from build123d import *

# Parameters (mm, degrees)
SKETCH1_W           = 260
SKETCH1_H           = 150
BOSS_EXTRUDE1_DEPTH = 15
SKETCH3_R           = 5
CUT_EXTRUDE1_DEPTH  = 16
SKETCH4_R           = 5
CUT_EXTRUDE2_DEPTH  = 16


with BuildPart() as part:
    # Sketch1 → Boss-Extrude1 (new body)
    with BuildSketch(Plane(origin=(0, 0, 0), x_dir=(0, 0, -1), z_dir=(1, 0, 0))):
        Rectangle(SKETCH1_W, SKETCH1_H)
    extrude(amount=BOSS_EXTRUDE1_DEPTH)

    # Sketch3 → Cut-Extrude1 (cut, through all)
    with BuildSketch(Plane.ZY):
        with Locations((0, 55)):
            Circle(SKETCH3_R)
    extrude(amount=-CUT_EXTRUDE1_DEPTH, mode=Mode.SUBTRACT)

    # Sketch4 → Cut-Extrude2 (cut, through all)
    with BuildSketch(Plane.ZY):
        with Locations((-120, 55)):
            Circle(SKETCH4_R)
        with Locations((-117.956771962, 32.950057862)):
            Circle(SKETCH4_R)
        with Locations((-111.896667529, 11.651000058)):
            Circle(SKETCH4_R)
        with Locations((-102.026056288, -8.171859545)):
            Circle(SKETCH4_R)
        with Locations((-88.681070066, -25.843477238)):
            Circle(SKETCH4_R)
        with Locations((-72.316156366, -40.762067274)):
            Circle(SKETCH4_R)
        with Locations((-53.488602693, -52.419594963)):
            Circle(SKETCH4_R)
        with Locations((-32.839558809, -60.419077181)):
            Circle(SKETCH4_R)
        with Locations((-11.072203136, -64.488101155)):
            Circle(SKETCH4_R)
        with Locations((11.072203136, -64.488101155)):
            Circle(SKETCH4_R)
        with Locations((32.839558809, -60.419077181)):
            Circle(SKETCH4_R)
        with Locations((53.488602693, -52.419594963)):
            Circle(SKETCH4_R)
        with Locations((72.316156366, -40.762067274)):
            Circle(SKETCH4_R)
        with Locations((88.681070066, -25.843477238)):
            Circle(SKETCH4_R)
        with Locations((102.026056288, -8.171859545)):
            Circle(SKETCH4_R)
        with Locations((111.896667529, 11.651000058)):
            Circle(SKETCH4_R)
        with Locations((117.956771962, 32.950057862)):
            Circle(SKETCH4_R)
        with Locations((120, 55)):
            Circle(SKETCH4_R)
    extrude(amount=-CUT_EXTRUDE2_DEPTH, mode=Mode.SUBTRACT)


solid = part.part
Geometry check sheet. Reference: the model listing, model coordinates, mm. Round coordinates to 2 decimals unless told otherwise and drop trailing zeros. Loops run counter-clockwise (first coordinate to the right, second up) from the corner with the lowest first, then second, coordinate; pieces in that order, holes last.
Item 1: Cross-section at D-D on x = 2.5. Count the separate pieces of the cut face and the enclosed holes in it, then the cut area to 3 significant figures.
Item 2: Cross-section at C-C on z = 0. Record the boundary of the cut face in (x, y), then the cut area to 3 significant figures.
Item 3: Gauge pin test, flat end, axial feed: pin 1 (11.5 mm diameter, centred on y = -40.76, z = -72.32, fed in from -X). Record the tip position at first contact, or that the pin passes through.
Item 4: Cross-section at B-B on z = -120. Record the boundary of the cut face in (x, y), then the cut area to 3 significant figures.
Item 5: Thickness scan on line 1 (Z direction, x = 4.5, y = 12); line 2 (Z direction, x = 6.5, y = -41); line 3 (Y direction, x = 1.5, z = 116.5). Record the ranges inside material, lowest first.
Item 6: Mould release check, pull along Z, two halves, no side actions. Record for faces 1 (the cylindrical face through (7.4, -69.37, 9.99)), 2 (the flat face through (7, -1, -130)), 3 (the flat face through (7, 75, 2)), 4 (the cylindrical face through (7.395, 59.957, -0.651)): pulls with the +Z half, pulls with the -Z half, needs draft (parallel to the pull), parting line crosses it, or undercut.
Item 7: Cross-section at A-A on y = 55. Record the boundary of the cut face in (x, z), then the cut area to 3 significant figures.
Answer sheet:
1. separate pieces: 1
1. enclosed holes: 19
1. area: 37,500 mm2
2. outline: (0, -75) - (15, -75) - (15, 50) - (0, 50) - close; (0, 60) - (15, 60) - (15, 75) - (0, 75) - close
2. area: 2,100 mm2
3. pin 1: stops at x = 0
4. outline: (0, -75) - (15, -75) - (15, 28.39) - (0, 28.39) - close; (0, 37.51) - (15, 37.51) - (15, 50) - (0, 50) - close; (0, 60) - (15, 60) - (15, 75) - (0, 75) - close
4. area: 1,960 mm2
5. line 1: z = -130 to -116.88, -106.91 to 106.91, 116.88 to 130
5. line 2: z = -130 to -77.31, -67.32 to 67.32, 77.31 to 130
5. line 3: y = -75 to 9.7, 13.6 to 28.17, 37.73 to 51.43, 58.57 to 75
6. face 1: undercut
6. face 2: pulls with the -Z half
6. face 3: needs draft
6. face 4: undercut
7. outline: (0, -130) - (15, -130) - (15, -125) - (0, -125) - close; (0, -115) - (15, -115) - (15, -5) - (0, -5) - close; (0, 5) - (15, 5) - (15, 115) - (0, 115) - close; (0, 125) - (15, 125) - (15, 130) - (0, 130) - close
7. area: 3,450 mm2
